Input: part model. Units: mm. Frame: model coordinates. A direction names the side the tool comes from. Round coordinates to 2 decimals unless told otherwise and drop trailing zeros. Write each loop counter-clockwise with the first axis right and the second up, starting at its lowest first coordinate (ties: lowest second). Pieces come first, ordered by that corner, then holes. Notation, with made-up numbers: (49, -37) -> (78, -37) arc R24 cw to (78, -6) -> close; hole circle Ø2 at (62, 80). An arc over 180 degrees is marked (long way). Write item = value, one per line.
```python
from build123d import *

# Parameters (mm, degrees)
PAD_DEPTH     = 12
POCKET_DEPTH  = 12.001
CHAMFER_ANGLE = 20
CHAMFER_SIZE  = 10


with BuildPart() as part:
    # Sketch → Pad (new body)
    with BuildSketch(Plane.XY):
        Polygon((0, 495), (165, 495), (165, 0), (0, 0), (0, 247.5), align=None)
    extrude(amount=PAD_DEPTH)

    # Sketch001 (on Face7 of Pad) → Pocket (cut, through all)
    with BuildSketch(Plane.XY.offset(12)):
        Polygon((45.608967, 259.905869), (28.476261, 245.880386), (45.608967, 231.854903), (45.608967, 241.205225), (54.959289, 241.205225), (54.959289, 250.555547), (45.608967, 250.555547), align=None)
    extrude(amount=-POCKET_DEPTH, mode=Mode.SUBTRACT)

    # Chamfer
    chamfer_edges = [part.edges().sort_by_distance(p)[0] for p in [
        (165, 247.5, 0),
    ]]
    chamfer_side = part.faces().sort_by_distance((165, 247.5, 6))[0]
    chamfer(chamfer_edges, length=CHAMFER_SIZE, angle=CHAMFER_ANGLE, reference=chamfer_side)


solid = part.part
```
1) Draft query along X for faces 1 (the face through (36.92, 238.97, 6.08)), 2 (the face through (81, 495, 6)), 3 (the face through (45.609, 255, 6)), 4 (the face through (163.155, 250.965, 4.93)). Return one class per face: +X half, -X half, draft (parallel to the pull), parting line (faces both ways), or undercut.
Solutions:
face_1 = undercut
face_2 = draft
face_3 = undercut
face_4 = +X half
2) Cut plane A-A (x = 40.5). Return the cut outline in (y, z).
Solutions:
outline = (0, 0) -> (236.04, 0) -> (236.04, 12) -> (0, 12) -> close; (255.72, 0) -> (495, 0) -> (495, 12) -> (255.72, 12) -> close
3) Cut plane B-B (z = 2). Return the cut outline in (x, y), and give its area (3 significant figures).
Solutions:
outline = (0, 0) -> (162.09, 0) -> (162.09, 495) -> (0, 495) -> close; hole (28.48, 245.88) -> (45.61, 231.85) -> (45.61, 241.21) -> (54.96, 241.21) -> (54.96, 250.56) -> (45.61, 250.56) -> (45.61, 259.91) -> close
area = 79,900 mm^2
4) Access query for faces 5 (the face through (50, 241.205, 6)), 6 (the face through (84, 251, 12)). Directions: +Z, -Z, +X, -X, +Y, -Y. A direction counts if a zero-diameter tool reaches every point of the face in a straight line with its end or side. Return the directions, or none.
Solutions:
face_5 = +Z, -Z
face_6 = +Z, +X, -X, +Y, -Y
5) First-contact query: P1, Ø5, axis at y = 148, z = 5, coming from the +X side. Flat tip, straight axial feed; report the tip coordinate or a pass-through.
Solutions:
P1 = 164.09
6) Line query: L1, parallel to X at y = 125, z = 4.75; L2, parallel to X at y = 167.5, z = 5.5. Output: solid intervals per line, ascending. Write a range as from..to.
Solutions:
L1 = 0..163.09
L2 = 0..163.36
